Work out the finished part from the listing and answer in its coordinate system (mm). A direction names the side the tool comes from. Coordinates: 2 decimals unless noted, no trailing zeros. Loops run counter-clockwise (first coordinate to the right, second up) from the corner with the lowest first, then second, coordinate; pieces in that order, holes last. Notation, with made-up numbers: (89, 29.25) -> (135, 29.25) arc R16 cw to (135, 42.25) -> close; hole circle Ø8 at (-33.75, 77.25). An arc over 180 degrees is marked (long way). Use a Markdown table: item, result.
from build123d import *

# Parameters (mm, degrees)
SKETCH_2_W          = 147
SKETCH_2_H          = 40
EXTRUDE_1_DEPTH     = 1.5
SKETCH_3_R          = 1.75
CUT_EXTRUDE_1_DEPTH = 10
SKETCH_4_W          = 8.5
SKETCH_4_H          = 30
SKETCH_4_W_2        = 6
SKETCH_4_W_3        = 7.5
CUT_EXTRUDE_2_DEPTH = 10
FILLET_1_R          = 3


with BuildPart() as part:
    # 草图2 → 凸台-拉伸1 (new body)
    with BuildSketch(Plane(origin=(0, 0, 0), x_dir=(1, 0, 0), z_dir=(0, 1, 0))):
        Rectangle(SKETCH_2_W, SKETCH_2_H)
    extrude(amount=EXTRUDE_1_DEPTH)

    # 草图3 → 切除-拉伸1 (cut)
    with BuildSketch(Plane.XZ):
        with Locations(Location((70.5, 15, 0), (0, 0, 270))):
            Circle(SKETCH_3_R)
        with Locations(Location((70.5, -5, 0), (0, 0, 270))):
            Circle(SKETCH_3_R)
        with Locations(Location((-70.5, 15, 0), (0, 0, 270))):
            Circle(SKETCH_3_R)
        with Locations(Location((-70.5, -5, 0), (0, 0, 270))):
            Circle(SKETCH_3_R)
    extrude(amount=-CUT_EXTRUDE_1_DEPTH, mode=Mode.SUBTRACT)

    # 草图4 → 切除-拉伸2 (cut)
    with BuildSketch(Plane(origin=(0, 1.5, 0), x_dir=(1, 0, 0), z_dir=(0, 1, 0))):
        with Locations((-59.25, 0)):
            Rectangle(SKETCH_4_W, SKETCH_4_H)
        with Locations((-49, 0)):
            Rectangle(SKETCH_4_W_2, SKETCH_4_H)
        with Locations((-40, 0)):
            Rectangle(SKETCH_4_W_2, SKETCH_4_H)
        with Locations((-31, 0)):
            Rectangle(SKETCH_4_W_2, SKETCH_4_H)
        with Locations((-22, 0)):
            Rectangle(SKETCH_4_W_2, SKETCH_4_H)
        with Locations((-13, 0)):
            Rectangle(SKETCH_4_W_2, SKETCH_4_H)
        with Locations((-4, 0)):
            Rectangle(SKETCH_4_W_2, SKETCH_4_H)
        with Locations((5, 0)):
            Rectangle(SKETCH_4_W_2, SKETCH_4_H)
        with Locations((14, 0)):
            Rectangle(SKETCH_4_W_2, SKETCH_4_H)
        with Locations((23, 0)):
            Rectangle(SKETCH_4_W_2, SKETCH_4_H)
        with Locations((32, 0)):
            Rectangle(SKETCH_4_W_2, SKETCH_4_H)
        with Locations((41, 0)):
            Rectangle(SKETCH_4_W_2, SKETCH_4_H)
        with Locations((50, 0)):
            Rectangle(SKETCH_4_W_2, SKETCH_4_H)
        with Locations((59.75, 0)):
            Rectangle(SKETCH_4_W_3, SKETCH_4_H)
    extrude(amount=-CUT_EXTRUDE_2_DEPTH, mode=Mode.SUBTRACT)

    # 圆角1
    fillet_1_edges = [part.edges().sort_by_distance(p)[0] for p in [
        (-52, 0.75, -15),
        (-46, 0.75, -15),
        (-37, 0.75, 15),
        (-43, 0.75, 15),
        (-43, 0.75, -15),
        (-37, 0.75, -15),
        (-28, 0.75, 15),
        (-34, 0.75, 15),
        (-34, 0.75, -15),
        (-28, 0.75, -15),
        (-19, 0.75, 15),
        (-25, 0.75, 15),
        (-25, 0.75, -15),
        (-19, 0.75, -15),
        (-10, 0.75, 15),
        (-16, 0.75, 15),
        (-16, 0.75, -15),
        (-10, 0.75, -15),
        (-1, 0.75, 15),
        (-7, 0.75, 15),
        (-7, 0.75, -15),
        (-1, 0.75, -15),
        (8, 0.75, 15),
        (2, 0.75, 15),
        (2, 0.75, -15),
        (8, 0.75, -15),
        (17, 0.75, 15),
        (11, 0.75, 15),
        (11, 0.75, -15),
        (17, 0.75, -15),
        (26, 0.75, 15),
        (20, 0.75, 15),
        (20, 0.75, -15),
        (26, 0.75, -15),
        (35, 0.75, 15),
        (29, 0.75, 15),
        (29, 0.75, -15),
        (35, 0.75, -15),
        (44, 0.75, 15),
        (38, 0.75, 15),
        (38, 0.75, -15),
        (44, 0.75, -15),
        (53, 0.75, 15),
        (47, 0.75, 15),
        (47, 0.75, -15),
        (53, 0.75, -15),
        (56, 0.75, 15),
        (56, 0.75, -15),
        (63.5, 0.75, -15),
        (63.5, 0.75, 15),
        (-55, 0.75, 15),
        (-63.5, 0.75, 15),
        (-63.5, 0.75, -15),
        (-55, 0.75, -15),
        (-46, 0.75, 15),
        (-52, 0.75, 15),
    ]]
    fillet(fillet_1_edges, radius=FILLET_1_R - 0.0001)  # a hair under: the kernel refuses the full size


solid = part.part
Q1. Section A-A on x = -70.5 is taken. Determine the outline of the cut face in (y, z), and give its area (3 significant figures).
Solved:
| item | result |
|---|---|
| outline | (0, -20) -> (1.5, -20) -> (1.5, -6.75) -> (0, -6.75) -> close; (0, -3.25) -> (1.5, -3.25) -> (1.5, 13.25) -> (0, 13.25) -> close; (0, 16.75) -> (1.5, 16.75) -> (1.5, 20) -> (0, 20) -> close |
| area | 49.5 mm² |
Q2. For faces 1 (the cylindrical face through (34.14, 0.74, -14.1)), 2 (the flat face through (-17, 1.5, 0)), determine the directions among +Z, -Z, +X, -X, +Y, -Y from which every point of the face is accessible in a straight line to the end or side of a thin tool.
Solved:
| item | result |
|---|---|
| face 1 | +Y, -Y |
| face 2 | +Z, -Z, +X, -X, +Y |
Q3. Given pin 1 Ø2 at (x, z) = (-56.5, 11) entering from +Y, flat-ended and moving along its own axis, determine where the tip first touches the part or whether it passes through.
Solved:
| item | result |
|---|---|
| pin 1 | through |
Q4. Section D-D on x = -50.5 is taken. Determine the outline of the cut face in (y, z).
Solved:
| item | result |
|---|---|
| outline | (0, -20) -> (1.5, -20) -> (1.5, -14.6) -> (0, -14.6) -> close; (0, 14.6) -> (1.5, 14.6) -> (1.5, 20) -> (0, 20) -> close |
Q5. Consider line 1 (Z direction, x = 70.5, y = 0.45); line 2 (Z direction, x = -58, y = 0.85); line 3 (X direction, y = 0.7, z = 16). Determine where each line is inside the solid, lowest interval first. Write a range as [from, to].
Solved:
| item | result |
|---|---|
| line 1 | [-20, -6.75], [-3.25, 13.25], [16.75, 20] |
| line 2 | [-20, -15], [15, 20] |
| line 3 | [-73.5, -71.94], [-69.06, 69.06], [71.94, 73.5] |
Q6. Section B-B on z = 1 is taken. State how many separate pieces and enclosed holes the cut face has, and give its area (3 significant figures).
Solved:
| item | result |
|---|---|
| separate pieces | 15 |
| enclosed holes | 0 |
| area | 88.5 mm² |
Q7. Determine the mould class of faces 3 (the cylindrical face through (-6.1, 0.74, 14.14)), 4 (the flat face through (-17, 0, 0)) for opening direction Z: pulls with the +Z half, pulls with the -Z half, needs draft (parallel to the pull), parting line crosses it, or undercut.
Solved:
| item | result |
|---|---|
| face 3 | undercut |
| face 4 | needs draft |
